For this review, take the finished solid that the model builds, in its own axes (mm). A direction names the side the tool comes from. Give positions to 0.01 mm unless a question says otherwise; leave off trailing zeros. Loops run counter-clockwise (first coordinate to the right, second up) from the corner with the lowest first, then second, coordinate; pieces in that order, holes last. Notation, with made-up numbers: (-9.75, 32.5) - (-0.75, 32.5) arc R25 ccw to (-0.75, 45.5) - close; hole circle Ø8 at (87, 59.25). An arc over 180 degrees is marked (long way). Put each result on its own line as item: value.
from build123d import *

# Parameters (mm, degrees)
F0_R     = 10
F1_DEPTH = 2.5
F3_DEPTH = 2.501


with BuildPart() as f1:
    # F0 (on Top) → F1 (new body)
    with BuildSketch(Plane.XY):
        Circle(F0_R)
    extrude(amount=F1_DEPTH)

    # F2 (on face) → F3 (cut, through all)
    with BuildSketch(Plane.XY.offset(2.5)):
        Polygon((4.935878, 5.812861), (0, 1.671168), (-4.935878, 5.812861), (-4.935878, -5.373671), (-3.259804, -5.373671), (-3.259804, 2.218509), (0, -0.516791), (3.259804, 2.218509), (3.259804, -5.373671), (4.935878, -5.373671), align=None)
    extrude(amount=-F3_DEPTH, mode=Mode.SUBTRACT)


solid = f1.part
1) Draft analysis for pull direction Y (two halves, no side actions). For faces 1 (the face through (-2.17, -9.76, 1.23)), 2 (the face through (0, -2, 2.5)), 3 (the face through (2.5, 3.77, 1.27)), state which applies: pulls with the +Y half, pulls with the -Y half, needs draft (parallel to the pull), parting line crosses it, or undercut.
Geometry check:
face 1: parting line crosses it
face 2: needs draft
face 3: undercut
2) Wall thickness on line 1 (X direction, y = -0.75, z = 1.5); line 2 (X direction, y = -3, z = 2); line 3 (X direction, y = 1.5, z = 1.6): over which ranges is each line inside the solid? List them lowest first.
Geometry check:
line 1: x = -9.97 to -4.94, -3.26 to 3.26, 4.94 to 9.97
line 2: x = -9.54 to -4.94, -3.26 to 3.26, 4.94 to 9.54
line 3: x = -9.89 to -4.94, -3.26 to -2.4, 2.4 to 3.26, 4.94 to 9.89
3) Take a section at B-B on x = 1. State the section outline as (y, z) points.
Geometry check:
outline: (-9.95, 0) - (0.32, 0) - (0.32, 2.5) - (-9.95, 2.5) - close; (2.51, 0) - (9.95, 0) - (9.95, 2.5) - (2.51, 2.5) - close
4) For faces 4 (the face through (4.936, 0, 1)), 5 (the face through (0, -2, 0)), list the 3-axis set-ups (+Z, -Z, +X, -X, +Y, -Y) from which the entire face can be reached by the end or side of a thin tool; tool diameter is ignored.
Geometry check:
face 4: +Z, -Z
face 5: -Z, +X, -X, +Y, -Y
5) Take a section at C-C on y = -4.5. State the section outline as (x, z) points, and give its area (3 significant figures).
Geometry check:
outline: (-8.93, 0) - (-4.94, 0) - (-4.94, 2.5) - (-8.93, 2.5) - close; (-3.26, 0) - (3.26, 0) - (3.26, 2.5) - (-3.26, 2.5) - close; (4.94, 0) - (8.93, 0) - (8.93, 2.5) - (4.94, 2.5) - close
area: 36.3 mm²
6) Take a section at D-D on y = 0. State the section outline as (x, z) points.
Geometry check:
outline: (-10, 0) - (-4.94, 0) - (-4.94, 2.5) - (-10, 2.5) - close; (-3.26, 0) - (-0.62, 0) - (-0.62, 2.5) - (-3.26, 2.5) - close; (0.62, 0) - (3.26, 0) - (3.26, 2.5) - (0.62, 2.5) - close; (4.94, 0) - (10, 0) - (10, 2.5) - (4.94, 2.5) - close
7) Insertion check: pin 1 Ø0.8 at (y, z) = (-3, 2) entering from +X; pin 2 Ø1.5 at (y, z) = (4, 0.5) entering from +X; pin 3 Ø1.2 at (y, z) = (1.5, 1.5) entering from +X. Each pin has a flat end and moves straight along its axis. Give the tip position at first contact, or say it passes through.
Geometry check:
pin 1: stops at x = 9.66
pin 2: stops at x = 9.46
pin 3: stops at x = 9.96
8) Take a section at A-A on z = 2.05. State the section outline as (x, y) points, and give its area (3 significant figures).
Geometry check:
outline: circle Ø20 at (0, 0); hole (-4.94, -5.37) - (-3.26, -5.37) - (-3.26, 2.22) - (0, -0.52) - (3.26, 2.22) - (3.26, -5.37) - (4.94, -5.37) - (4.94, 5.81) - (0, 1.67) - (-4.94, 5.81) - close
area: 265 mm²
